from build123d import *

# Parameters (mm, degrees)
SKETCH1_R           = 1.65
BOSS_EXTRUDE1_DEPTH = 3.2
SKETCH2_W           = 4
SKETCH2_H           = 12
BOSS_EXTRUDE2_DEPTH = 3.2
FILLET1_R           = 1.5


with BuildPart() as part:
    # Sketch1 → Boss-Extrude1 (new body)
    with BuildSketch(Plane.XY):
        with BuildLine():
            Line((1.830127019, -31.504464167), (35.605117766, -51.004464167))
            Line((35.605117766, -51.004464167), (48.732545217, -54.648197122))
            ThreePointArc((48.732545217, -54.648197122), (49.6052046, -54.480696676), (50, -53.68462671))
            Line((50, -53.68462671), (50, 44))
            Line((50, 44), (48.060403212, 55))
            Line((48.060403212, 55), (46, 55))
            Line((46, 55), (0, -24.674337148))
            ThreePointArc((0, -24.674337148), (-0.499502113, -28.468432374), (1.830127019, -31.504464167))
        make_face()
        with Locations((38, -5)):
            Circle(SKETCH1_R, mode=Mode.SUBTRACT)
    extrude(amount=BOSS_EXTRUDE1_DEPTH)

    # Sketch2 → Boss-Extrude2 (add)
    with BuildSketch(Plane.XY.offset(3.2)):
        with Locations((52, 26)):
            Rectangle(SKETCH2_W, SKETCH2_H)
    extrude(amount=-BOSS_EXTRUDE2_DEPTH)

    # Fillet1
    fillet1_edges = [part.edges().sort_by_distance(p)[0] for p in [
        (54, 32, 1.6),
        (54, 20, 1.6),
    ]]
    fillet(fillet1_edges, radius=FILLET1_R)


solid = part.part
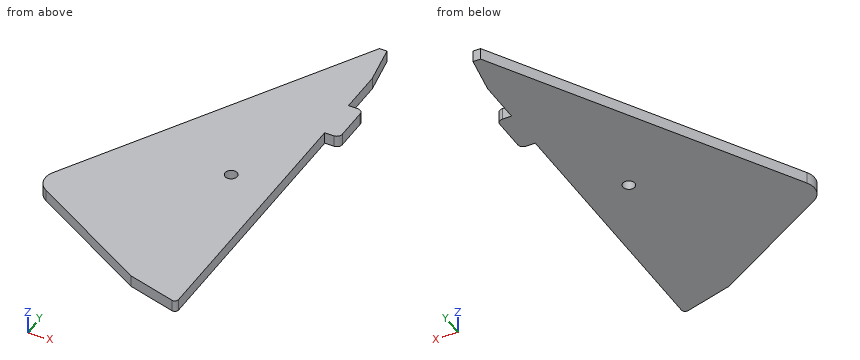
Here's how the part is built. I have some questions about the finished solid (model axes, mm). Round coordinates to 2 decimals unless told otherwise and drop trailing zeros. Write each loop counter-clockwise with the first axis right and the second up, starting at its lowest first coordinate (ties: lowest second). Pieces come first, ordered by that corner, then holes. Notation, with made-up numbers: (1.25, 10) -> (44.25, 10) arc R18 cw to (44.25, 37) -> close; hole circle Ø5 at (44, 29). An arc over 180 degrees is marked (long way). One line per item, written item: value.
1) Suppose I cut it at B-B on y = -5. List the corners of the cut face in (x, z) for me, plus the area to 3 significant figures.
Filled sheet:
outline: (11.36, 0) -> (36.35, 0) -> (36.35, 3.2) -> (11.36, 3.2) -> close; (39.65, 0) -> (50, 0) -> (50, 3.2) -> (39.65, 3.2) -> close
area: 113 mm2
2) Suppose I cut it at A-A on z = 2.45. List the corners of the cut face in (x, y) for me.
Filled sheet:
outline: (0, -24.67) arc R5 ccw to (1.83, -31.5) -> (35.61, -51) -> (48.73, -54.65) arc R1 ccw to (50, -53.68) -> (50, 20) -> (52.5, 20) arc R1.5 ccw to (54, 21.5) -> (54, 30.5) arc R1.5 ccw to (52.5, 32) -> (50, 32) -> (50, 44) -> (48.06, 55) -> (46, 55) -> close; hole circle Ø3.3 at (38, -5)
3) I'm going to push flat-ended pins straight in: pin 1 Ø1.2 at (x, z) = (51.5, 1.5) entering from -Y; pin 2 Ø1 at (y, z) = (-11, 1.5) entering from +X. Where does each tip first touch, or does it pass through?
Filled sheet:
pin 1: stops at y = 20
pin 2: stops at x = 50
4) Suppose I cut it at D-D on y = -40. List the corners of the cut face in (x, z) for me.
Filled sheet:
outline: (16.54, 0) -> (50, 0) -> (50, 3.2) -> (16.54, 3.2) -> close
5) If I drill on line 1 (Y direction, x = 39, z = 1.6); line 2 (Y direction, x = 38, z = 2.25); line 3 (X direction, y = 29.5, z = 2.25), over which ranges is the centre line in solid material (lowest first)? Write a range as [from, to].
Filled sheet:
line 1: y = [-51.95, -6.31], [-3.69, 42.88]
line 2: y = [-51.67, -6.65], [-3.35, 41.14]
line 3: x = [31.28, 54]
6) Suppose I cut it at C-C on x = 38. List the corners of the cut face in (y, z) for me, plus the area to 3 significant figures.
Filled sheet:
outline: (-51.67, 0) -> (-6.65, 0) -> (-6.65, 3.2) -> (-51.67, 3.2) -> close; (-3.35, 0) -> (41.14, 0) -> (41.14, 3.2) -> (-3.35, 3.2) -> close
area: 286 mm2
